```python
from build123d import *

# Parameters (mm, degrees)
ESQUISSE1_R                  = 30
ESQUISSE1_R_2                = 11
BOSS_EXTRU_1_DEPTH           = 6
ESQUISSE2_R                  = 30
BOSS_EXTRU_2_DEPTH           = 2
ENL_V_MAT_EXTRU_1_DEPTH      = 1
ENL_V_MAT_EXTRU_1_DEPTH_BACK = 1
ESQUISSE3_R                  = 30
ESQUISSE3_R_2                = 29
ESQUISSE4_R                  = 4.5
AJOURAGE_DEPTH               = 44.17406629


with BuildPart() as part:
    # Esquisse1 → Boss.-Extru.1 (new body)
    with BuildSketch(Plane.XY):
        Circle(ESQUISSE1_R)
        Circle(ESQUISSE1_R_2, mode=Mode.SUBTRACT)
    extrude(amount=BOSS_EXTRU_1_DEPTH)

    # Esquisse2 → Boss.-Extru.2 (add)
    with BuildSketch(Plane.XY.offset(6)):
        Circle(ESQUISSE2_R)
    extrude(amount=BOSS_EXTRU_2_DEPTH)

    # Esquisse3 → Enlèv. mat.-Extru.1 (cut, two sides: drawn at the far end of the back side and taken through both)
    with BuildSketch(Plane.XY.offset(4).offset(-ENL_V_MAT_EXTRU_1_DEPTH_BACK)):
        Circle(ESQUISSE3_R)
        Circle(ESQUISSE3_R_2, mode=Mode.SUBTRACT)
    extrude(amount=ENL_V_MAT_EXTRU_1_DEPTH + ENL_V_MAT_EXTRU_1_DEPTH_BACK, mode=Mode.SUBTRACT)

    # Esquisse4 → Ajourage (cut, through all)
    with BuildSketch(Plane.XY.offset(8)):
        with Locations((21, 0)):
            Circle(ESQUISSE4_R)
        with Locations((10.5, 18.186533479)):
            Circle(ESQUISSE4_R)
        with Locations((-10.5, 18.186533479)):
            Circle(ESQUISSE4_R)
        with Locations((-21, 0)):
            Circle(ESQUISSE4_R)
        with Locations((-10.5, -18.186533479)):
            Circle(ESQUISSE4_R)
        with Locations((10.5, -18.186533479)):
            Circle(ESQUISSE4_R)
    extrude(amount=-AJOURAGE_DEPTH, mode=Mode.SUBTRACT)


solid = part.part
```
Source: CAD feature listing. Evaluate the final solid. Frame: model axes, mm. A direction names the side the tool comes from. Coordinates: 2 decimals unless noted, no trailing zeros. Loops run counter-clockwise (first coordinate to the right, second up) from the corner with the lowest first, then second, coordinate; pieces in that order, holes last. Notation, with made-up numbers: M -39.75,3 L 1.25,3 A8 ccw 1.25,16 Z; hole C 41,70 d7. An arc over 180 degrees is marked long. Put each result on its own line as item: value. Start each with the question number.
1) Cut plane D-D on z = 2.25. Return the cut outline in (x, y).
2) Cut plane A-A on y = 0. Return the cut outline in (x, z), then the cut area to 3 significant figures.
3) Cut plane B-B on x = 22.5. Return the cut outline in (y, z), then the cut area to 3 significant figures.
4) Pull-direction query (Z, two-part tool) for faces 1 (the face through (-16, 25, 5)), 2 (the face through (13, 0, 0)), 3 (the face through (-16, 25, 3)), 4 (the face through (9.914, 22.648, 4.056)); classes: pulls with the +Z half, pulls with the -Z half, needs draft (parallel to the pull), parting line crosses it, or undercut.
5) Contact query for flat-ended pins moving along their axis: pin 1 Ø4 at (y, z) = (15.5, 1) entering from -X; pin 2 Ø1 at (x, z) = (21, 5) entering from -Y; pin 3 Ø7 at (x, y) = (-21, 0) entering from +Z; pin 4 Ø6.5 at (x, y) = (-3.5, 2) entering from -Z. Output: stop coordinate, or through.
6) Cut plane C-C on x = -3. Return the cut outline in (y, z).
7) Ray query, L1, parallel to X at y = -18, z = 2; L2, parallel to Y at x = -14, z = 6.5; L3, parallel to X at y = -19, z = 6.25. Return the intervals inside material, ascending. Write a range as from..to.
8) Reachability of faces 5 (the face through (-2.38, -10.74, 2.96)), 6 (the face through (13.38, -25.73, 3.99)), 7 (the face through (-29.97, 1.32, 1.48)) from +Z, -Z, +X, -X, +Y, -Y: full face, straight path, thin tool, end or side. Return the list, or none.
The answers:
1. outline: C 0,0 d60; hole C -21,0 d9; hole C -10.5,-18.19 d9; hole C -10.5,18.19 d9; hole C 0,0 d22; hole C 10.5,-18.19 d9; hole C 10.5,18.19 d9; hole C 21,0 d9
2. outline: M -30,0 L -25.5,0 L -25.5,8 L -30,8 L -30,5 L -29,5 L -29,3 L -30,3 Z; M -16.5,0 L -11,0 L -11,6 L 11,6 L 11,0 L 16.5,0 L 16.5,8 L -16.5,8 Z; M 25.5,0 L 30,0 L 30,3 L 29,3 L 29,5 L 30,5 L 30,8 L 25.5,8 Z
2. area: 200 mm²
3. outline: M -19.84,0 L -4.24,0 L -4.24,8 L -19.84,8 L -19.84,5 L -18.3,5 L -18.3,3 L -19.84,3 Z; M 4.24,0 L 19.84,0 L 19.84,3 L 18.3,3 L 18.3,5 L 19.84,5 L 19.84,8 L 4.24,8 Z
3. area: 243 mm²
4. face 1: undercut
4. face 2: pulls with the -Z half
4. face 3: undercut
4. face 4: needs draft
5. pin 1: stops at x = -26.79
5. pin 2: stops at y = -21.9
5. pin 3: passes through
5. pin 4: stops at z = 6
6. outline: M -29.85,0 L -10.58,0 L -10.58,6 L 10.58,6 L 10.58,0 L 29.85,0 L 29.85,3 L 28.84,3 L 28.84,5 L 29.85,5 L 29.85,8 L -29.85,8 L -29.85,5 L -28.84,5 L -28.84,3 L -29.85,3 Z
7. L1: x = -24..-15, -6..6, 15..24
7. L2: y = -26.53..-21.01, -15.36..15.36, 21.01..26.53
7. L3: x = -23.22..-14.93, -6.07..6.07, 14.93..23.22
8. face 5: -Z
8. face 6: none
8. face 7: +Z, -Z
